For this review, use the dimensioned drawing (mm, ordinates from the lowest corner) and the shaded views. A direction names the side the tool comes from. Round coordinates to 2 decimals unless told otherwise and drop trailing zeros. Order: outer loops, then holes, each group sorted by start corner. A loop starts at its lowest first (then second) coordinate and runs counter-clockwise, first axis right, second up. Notation, with made-up numbers: (-31, 77.25) -> (21, 77.25) arc R27 ccw to (21, 113.25) -> close; hole circle Ø3 at (-35, 70). An arc over 180 degrees is marked (long way). Answer in a Markdown table with one row per item.
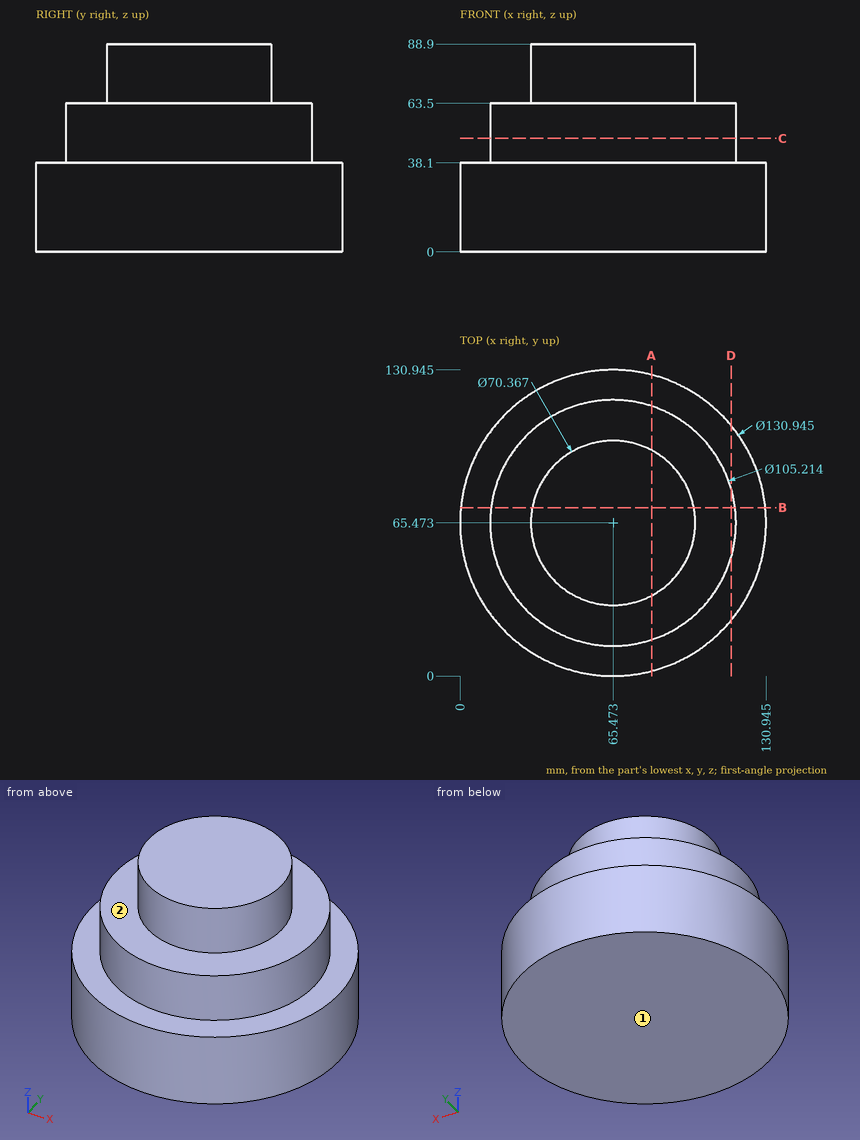
Q1. Clearance check with flat-ended pins moving along their axes: pin 1 Ø2 at (y, z) = (26, 24) entering from +X; pin 2 Ø5 at (x, y) = (14, 107.5) entering from -Z; pin 3 Ø1 at (x, y) = (95.5, 85.5) entering from +Z; pin 4 Ø4 at (x, z) = (22.5, 61.5) entering from -Y (1 decimal). State where each tip first meets the part, or that it passes through.
Answer key:
| item | result |
|---|---|
| pin 1 | stops at x = 118.45 |
| pin 2 | stops at z = 0 |
| pin 3 | stops at z = 63.5 |
| pin 4 | stops at y = 32.5 |
Q2. To check wall thickness, follow probe 1 along Z at (x, y) = (111, 100); probe 2 along Z at (x, y) = (34, 34); probe 3 along X at (y, z) = (64, 28). State the ranges of each line that lie inside material, in increasing order.
Answer key:
| item | result |
|---|---|
| probe 1 | z = 0 to 38.1 |
| probe 2 | z = 0 to 63.5 |
| probe 3 | x = 0.02 to 130.93 |
Q3. Take a section at D-D, the plane x = 116. Write out the cut boundary in (y, z) (1 decimal), then the cut area to 3 significant figures.
Answer key:
| item | result |
|---|---|
| outline | (23.8, 0) -> (107.1, 0) -> (107.1, 38.1) -> (80.1, 38.1) -> (80.1, 63.5) -> (50.8, 63.5) -> (50.8, 38.1) -> (23.8, 38.1) -> close |
| area | 3,920 mm^2 |
Q4. Take a section at A-A, the plane x = 82. Write out the cut boundary in (y, z) (1 decimal).
Answer key:
| item | result |
|---|---|
| outline | (2.1, 0) -> (128.8, 0) -> (128.8, 38.1) -> (115.4, 38.1) -> (115.4, 63.5) -> (96.5, 63.5) -> (96.5, 88.9) -> (34.4, 88.9) -> (34.4, 63.5) -> (15.5, 63.5) -> (15.5, 38.1) -> (2.1, 38.1) -> close |
Q5. Take a section at B-B, the plane y = 72. Write out the cut boundary in (x, z) (1 decimal), then the cut area to 3 significant figures.
Answer key:
| item | result |
|---|---|
| outline | (0.3, 0) -> (130.6, 0) -> (130.6, 38.1) -> (117.7, 38.1) -> (117.7, 63.5) -> (100, 63.5) -> (100, 88.9) -> (30.9, 88.9) -> (30.9, 63.5) -> (13.3, 63.5) -> (13.3, 38.1) -> (0.3, 38.1) -> close |
| area | 9,370 mm^2 |
Q6. Tool access review of the marked faces 1 and 2: name each direction out of +Z, -Z, +X, -X, +Y, -Y from which nothing blocks a thin tool from reaching the whole face with its end or side.
Answer key:
| item | result |
|---|---|
| face 1 | -Z, +X, -X, +Y, -Y |
| face 2 | +Z |
Q7. Take a section at C-C, the plane z = 48.5. Write out the cut boundary in (x, y).
Answer key:
| item | result |
|---|---|
| outline | circle Ø105.21 at (65.47, 65.47) |
